Check sheet for the modelled part. Datum: model origin and axes. Units: mm. A direction names the side the tool comes from. Give positions to 0.01 mm unless a question says otherwise; leave off trailing zeros. Loops run counter-clockwise (first coordinate to the right, second up) from the corner with the lowest first, then second, coordinate; pieces in that order, holes last. Notation, with made-up numbers: M -20.75,-40 L -16.75,-40 A17 ccw -16.75,-20 Z; hole C 60,28 d3. An arc over 180 degrees is marked long. Write each question's results on one line, items separated by ' | '. Start each with the question number.
1. Sectioned sample at A-A on y = 9.25. Record the cut outline in (x, z), and give its area (3 significant figures).
2. Go/stop test with flat-tipped pins: pin 1 (5.5 mm diameter, centred on y = 8, z = 4, fed in from -X); pin 2 (7.5 mm diameter, centred on y = -11, z = 3.5, fed in from +X); pin 3 (14 mm diameter, centred on x = 0, y = -1.5, fed in from -Z). Record where each tip stops, or that it passes through.
3. Sectioned sample at B-B on x = -10.75. Record the cut outline in (y, z), and give its area (3 significant figures).
4. Sectioned sample at C-C on z = 2.5. Give the number of separate pieces and of enclosed holes in the cut face, and give its area (3 significant figures).
5. Tool access check on faces 1 (the flat face through (12, 8, 3)), 2 (the flat face through (-12, -8, 3)), 3 (the cylindrical face through (9.82, -8.78, 12.92)), 4 (the cylindrical face through (9.91, 8.71, 12.92)), 5 (the flat face through (12, -8, 3)). Record the directions out of +Z, -Z, +X, -X, +Y, -Y that give a thin tool (end or side, any length) a straight path to the whole face; none if there is none.
6. Draft check along Z on faces 6 (the flat face through (0, -11, 7)), 7 (the flat face through (0, 5, 11)), 8 (the cylindrical face through (0.17, -11.66, 3.87)), 9 (the cylindrical face through (-9.91, -8.71, 12.92)). Enter one of: pulls with the +Z half, pulls with the -Z half, needs draft (parallel to the pull), parting line crosses it, or undercut.
7. Material ranges on line 1 along Y through (x, z) = (-0.25, 3.5); line 2 along Y through (x, z) = (0, 12.2); line 3 along Y through (x, z) = (-3.75, 3.5), recorded low to high.
```python
from build123d import *

# Parameters (mm, degrees)
SKETCH1_W            = 24
SKETCH1_H            = 3.5
SKETCH1_R            = 8.1
BOSS_EXTRUDE1_DEPTH  = 7
BOSS_EXTRUDE2_START  = 7
SKETCH1_3_R          = 8.1
BOSS_EXTRUDE2_DEPTH  = 12
M3_CLEARANCE_HOLE1_D = 3.4
FILLET1_R            = 6
BOSS_EXTRUDE3_START  = 11
SKETCH1_4_R          = 8.1
SKETCH1_4_R_2        = 6
BOSS_EXTRUDE3_DEPTH  = 2


with BuildPart() as part:
    # Sketch1 → Boss-Extrude1 (new body)
    # profile 1 of 5: a face of its own
    with BuildSketch(Plane.XY):
        with Locations((0, 11.75)):
            Rectangle(SKETCH1_W, SKETCH1_H)
    # profile 2 of 5: a face of its own
    with BuildSketch(Plane.XY):
        with BuildLine():
            Line((-10, 10), (-12, 10))
            Line((-12, 10), (-12, 5.5))
            add(Edge.make_bspline(
                [(-12, 5.5), (-16.208168435, -1.452739177), (-12, -5.5)],
                knots=[0, 0, 0, 0.703674115, 0.703674115, 0.703674115], degree=2))
            Line((-12, -5.5), (-12, -10))
            Line((-12, -10), (-10, -10))
            Line((-10, -10), (-10, -5.5))
            add(Edge.make_bspline(
                [(-10, 5.5), (-13.144989471, -1.593519523), (-10, -5.5)],
                knots=[0, 0, 0, 0.703674115, 0.703674115, 0.703674115], degree=2))
            Line((-10, 5.5), (-10, 10))
        make_face()
    # profile 3 of 5: a face of its own
    with BuildSketch(Plane.XY):
        with BuildLine():
            Line((12, 5.5), (12, 10))
            Line((12, 10), (10, 10))
            Line((10, 10), (10, 5.5))
            add(Edge.make_bspline(
                [(10, 5.5), (13.144989471, -1.593519523), (10, -5.5)],
                knots=[0, 0, 0, 0.703674115, 0.703674115, 0.703674115], degree=2))
            Line((10, -5.5), (10, -10))
            Line((10, -10), (12, -10))
            Line((12, -10), (12, -5.5))
            add(Edge.make_bspline(
                [(12, 5.5), (16.208168435, -1.452739177), (12, -5.5)],
                knots=[0, 0, 0, 0.703674115, 0.703674115, 0.703674115], degree=2))
        make_face()
    # profile 4 of 5: a face of its own
    with BuildSketch(Plane.XY):
        with BuildLine():
            Line((-10, -10), (-12, -10))
            Line((-12, -10), (-12, -13.5))
            Line((-12, -13.5), (12, -13.5))
            Line((12, -13.5), (12, -10))
            Line((12, -10), (10, -10))
            Line((10, -10), (5.934098246, -10))
            add(Edge.make_bspline(
                [(5.934098246, -10), (5.478588927, -10.00932896), (0, -10)],
                knots=[0.968742805, 0.968742805, 0.968742805, 1, 1, 1], degree=2))
            Line((0, -10), (-10, -10))
        make_face()
    # profile 5 of 5: a face of its own
    with BuildSketch(Plane.XY):
        with BuildLine():
            Line((10, 10), (-10, 10))
            Line((-10, 10), (-10, 5.5))
            add(Edge.make_bspline(
                [(-10, 5.5), (-13.144989471, -1.593519523), (-10, -5.5)],
                knots=[0, 0, 0, 0.703674115, 0.703674115, 0.703674115], degree=2))
            Line((-10, -5.5), (-10, -10))
            Line((-10, -10), (0, -10))
            Line((0, -10), (5.934098246, -10))
            Line((5.934098246, -10), (10, -10))
            Line((10, -10), (10, -5.5))
            add(Edge.make_bspline(
                [(10, 5.5), (13.144989471, -1.593519523), (10, -5.5)],
                knots=[0, 0, 0, 0.703674115, 0.703674115, 0.703674115], degree=2))
            Line((10, 5.5), (10, 10))
        make_face()
        with Locations((0, -1.5)):
            Circle(SKETCH1_R, mode=Mode.SUBTRACT)
    extrude(amount=BOSS_EXTRUDE1_DEPTH)

    # Sketch1<3> → Boss-Extrude2 (add)
    with BuildSketch(Plane.XY.offset(BOSS_EXTRUDE2_START)):
        with BuildLine():
            Line((-12, 10), (-12, 5.5))
            add(Edge.make_bspline(
                [(-12, 5.5), (-16.208168435, -1.452739177), (-12, -5.5)],
                knots=[0, 0, 0, 0.703674115, 0.703674115, 0.703674115], degree=2))
            Line((-12, -5.5), (-12, -10))
            Line((-12, -10), (12, -10))
            Line((12, -10), (12, -5.5))
            add(Edge.make_bspline(
                [(12, 5.5), (16.208168435, -1.452739177), (12, -5.5)],
                knots=[0, 0, 0, 0.703674115, 0.703674115, 0.703674115], degree=2))
            Line((12, 5.5), (12, 10))
            Line((12, 10), (-12, 10))
        make_face()
        with Locations((0, -1.5)):
            Circle(SKETCH1_3_R, mode=Mode.SUBTRACT)
    extrude(amount=BOSS_EXTRUDE2_DEPTH)

    # M3 Clearance Hole1 (through all)
    with Locations(Plane.ZY.offset(12)):
        with Locations((3.5, 10), (3.5, -10)):
            Hole(M3_CLEARANCE_HOLE1_D / 2)

    # Fillet1
    # the kernel refuses this fillet: 6 mm, written as the material it takes off along each edge
    with BuildSketch(Plane(origin=(-12, 10, 7), x_dir=(1, 0, 0), z_dir=(0, 0, 1))) as fillet1_piece_1:
        with BuildLine():
            CenterArc((5.809475019, -6), FILLET1_R, 90, 75.522487814)
            Line((0, -4.5), (0, 0))
            Line((0, 0), (5.809475019, 0))
        make_face()
    extrude(amount=26.523687548, mode=Mode.SUBTRACT)
    with BuildSketch(Plane(origin=(12, 10, 7), x_dir=(0, -1, 0), z_dir=(0, 0, 1)), Plane(origin=(-12, -10, 7), x_dir=(0, 1, 0), z_dir=(0, 0, 1))) as fillet1_piece_2:
        with BuildLine():
            CenterArc((6, -5.809475019), FILLET1_R, 104.477512186, 75.522487814)
            Line((0, -5.809475019), (0, 0))
            Line((0, 0), (4.5, 0))
        make_face()
    extrude(amount=26.523687548, mode=Mode.SUBTRACT)
    with BuildSketch(Plane(origin=(12, -10, 7), x_dir=(0, 1, 0), z_dir=(0, 0, 1))) as fillet1_piece_3:
        with BuildLine():
            CenterArc((6, 5.809475019), FILLET1_R, 180, 75.522487814)
            Line((0, 5.809475019), (0, 0))
            Line((0, 0), (4.5, 0))
        make_face()
    extrude(amount=26.523687548, mode=Mode.SUBTRACT)

    # Sketch1<4> → Boss-Extrude3 (add)
    with BuildSketch(Plane.XY.offset(BOSS_EXTRUDE3_START)):
        with Locations((0, -1.5)):
            Circle(SKETCH1_4_R)
        with Locations((0, -1.5)):
            Circle(SKETCH1_4_R_2, mode=Mode.SUBTRACT)
    extrude(amount=BOSS_EXTRUDE3_DEPTH)

    # Fillet2: read off the stored shape, not the designer's step
    # Fillet2 outline → Fillet2 (revolve, cut)
    with BuildSketch(Plane.XZ.offset(1.5)):
        with BuildLine():
            ThreePointArc((10.1, 0), (8.685786438, 0.585786438), (8.1, 2))
            Line((8.1, 2), (8.1, 0))
            Line((8.1, 0), (10.1, 0))
        make_face()
    revolve(axis=Axis((0, -1.5, 0), (0, 0, 1)), mode=Mode.SUBTRACT)


solid = part.part
```
Output values:
1) outline: M -12,0 L 12,0 L 12,1.97 L -12,1.97 Z; M -12,5.03 L 12,5.03 L 12,7 L 9.1,7 L 9.1,19 L -9.1,19 L -9.1,7 L -12,7 Z | area: 313 mm2
2) pin 1: x = -12.15 | pin 2: x = 12 | pin 3: z = 11
3) outline: M -13.5,0 L 13.5,0 L 13.5,7 L 7.9,7 L 7.9,19 L -7.9,19 L -7.9,7 L -13.5,7 Z; hole C -10,3.5 d3.4; hole C 10,3.5 d3.4 | area: 360 mm2
4) separate pieces: 3 | enclosed holes: 0 | area: 346 mm2
5) face 1: +Z, -Z, +X, +Y | face 2: +Z, -Z, -X, -Y | face 3: +Z, +X, -Y | face 4: +Z, +X, +Y | face 5: +Z, -Z, +X, -Y
6) face 6: pulls with the +Z half | face 7: pulls with the -Z half | face 8: undercut | face 9: needs draft
7) line 1: -13.5 to -11.7, 6.6 to 8.3, 11.7 to 13.5 | line 2: -10 to -7.5, 4.5 to 10 | line 3: -13.5 to -11.7, 5.68 to 8.3, 11.7 to 13.5
